Here's how the part is built. I have some questions about the finished solid (model axes, mm). Coordinates: 2 decimals unless noted, no trailing zeros. Write each loop counter-clockwise with the first axis right and the second up, starting at its lowest first coordinate (ties: lowest second). Pieces come first, ordered by that corner, then holes.
Item 1: If I drill on line 1 (Y direction, x = 2.5, z = 1.85); line 2 (Y direction, x = 13.5, z = 1.6); line 3 (X direction, y = 2.5, z = 1.85), over which ranges is the centre line in solid material (lowest first)?
Item 2: If we section it at A-A (y = 75.5): Please give me the cut outline in (x, z).
Item 3: I'm going to push flat-ended pins straight in: pin 1 Ø1.5 at (x, z) = (9, 3) entering from +Y; pin 2 Ø3 at (x, y) = (2.5, 2.5) entering from +Z. Where does each tip first touch, or does it pass through?
Item 4: If we section it at C-C (y = 54): Please give me the cut outline in (x, z).
Item 5: If we section it at B-B (x = 13.5): Please give me the cut outline in (y, z).
Item 6: If we section it at D-D (z = 2.8): Please give me the cut outline in (x, y).
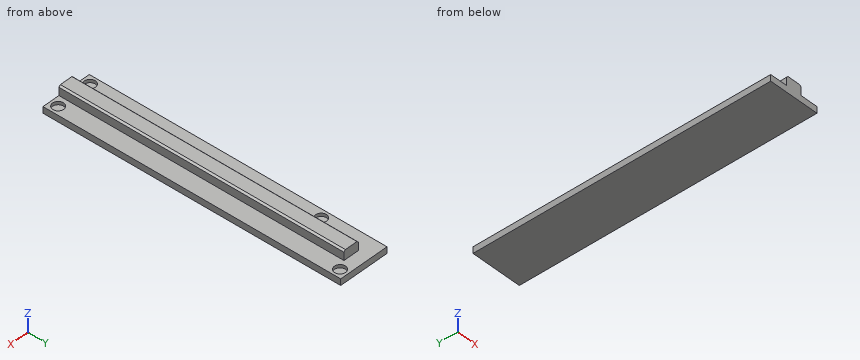
Autodesk Fusion 360 part; units mm, degrees
sketch "3D-printed conduit top outline" plane through (0, 0, 0) normal (0, 1, 0) x (1, 0, 0)
  line L0 (0, 0) -> (16, 0)
  line L1 (16, 0) -> (16, -2)
  line L2 (16, -2) -> (0, -2)
  line L3 (0, -2) -> (0, 0)
  dimension "d7" = 16
  dimension "d8" = 2
extrude "Extrude1" add sketch "3D-printed conduit top outline" along normal blind 94
sketch "Magnet holes" plane through (0, 0, 2) normal (0, 0, 1) x (-1, 0, 0)
  line L0 (0, 0) -> (-16, 0)
  line L1 (-16, 0) -> (-16, -94)
  line L2 (-16, -94) -> (0, -94)
  line L3 (0, -94) -> (0, 0)
  circle A0 centre (-2.5, -2.5) radius 2.5
  circle A1 centre (-13.5, -2.5) radius 2.5
  circle A2 centre (-2.5, -2.5) radius 1.75
  circle A3 centre (-13.5, -2.5) radius 1.75
  circle A4 centre (-2.5, -75.5) radius 1.75
  circle A5 centre (-2.5, -75.5) radius 2.5
  circle A6 centre (-13.5, -91.5) radius 2.5
  circle A7 centre (-13.5, -91.5) radius 1.75
  dimension "d11" = 5
  dimension "d12" = 5
  dimension "d13" = 3.5
  dimension "d14" = 3.5
  dimension "d17" = 0
  dimension "d18" = -73
  dimension "d32" = 0
  dimension "d33" = -89
extrude "Extrude4" cut sketch "Magnet holes" against normal blind 1 contours A2 | A3 | A4 | A7
sketch "Support rib" plane through (0, 0, 2) normal (0, 0, 1) x (-1, 0, 0)
  circle A0 centre (-13.5, -2.5) radius 1.75
  circle A1 centre (-2.5, -75.5) radius 1.75
  circle A2 centre (-2.5, -2.5) radius 1.75
  circle A3 centre (-13.5, -91.5) radius 1.75
  line L0 (0, 0) -> (-16, 0)
  line L1 (-16, 0) -> (-16, -94)
  line L2 (-16, -94) -> (0, -94)
  line L3 (0, -94) -> (0, 0)
  line L4 (-5.5, 0) -> (-10.5, 0)
  line L5 (-10.5, 0) -> (-10.5, -90)
  line L6 (-10.5, -90) -> (-5.5, -90)
  line L7 (-5.5, -90) -> (-5.5, 0)
  dimension "d36" = 5
  dimension "d37" = 5.5
  dimension "d38" = 5.5
  dimension "d39" = 4
extrude "Extrude3" add sketch "Support rib" along normal blind 3 contours L0 L4 L5 L6 L7
chamfer "Chamfer2" distance 0.5 angle 45 2 edges at (10.5, 45, 5) (5.5, 45, 5)
equation "conduit_length = 94 mm"
equation "conduit_width = 16 mm"
equation "conduit_wall_thickness = 2 mm"
equation "magnet_diameter = 3 mm"
equation "magnet_height = 1 mm"
equation "d7 = conduit_width"
equation "d8 = conduit_wall_thickness"
equation "d9 = conduit_length"
equation "d11 = magnet_diameter + 2 mm"
equation "d12 = magnet_diameter + 2 mm"
equation "d13 = magnet_diameter + 0.5 mm"
equation "d14 = magnet_diameter + 0.5 mm"
equation "d18 = -conduit_length + ( magnet_diameter + 2 mm ) + ( conduit_width )"
equation "rib_width = 5 mm"
equation "rib_height = 3 mm"
equation "d26 = rib_height"
equation "rib_chamfer = 0.5 mm"
equation "d33 = -conduit_length + ( magnet_diameter + 2 mm )"
equation "d36 = rib_width"
equation "d37 = ( conduit_width - rib_width ) / 2"
equation "d39 = 2 * conduit_wall_thickness"
equation "d40 = rib_chamfer"
Answer list:
1. line 1: y = 0 to 0.75, 4.25 to 73.75, 77.25 to 94
1. line 2: y = 0 to 0.75, 4.25 to 89.75, 93.25 to 94
1. line 3: x = 0 to 0.75, 4.25 to 11.75, 15.25 to 16
2. outline: (0, 0) - (16, 0) - (16, 2) - (10.5, 2) - (10.5, 4.5) - (10, 5) - (6, 5) - (5.5, 4.5) - (5.5, 2) - (4.25, 2) - (4.25, 1) - (0.75, 1) - (0.75, 2) - (0, 2) - close
3. pin 1: stops at y = 90
3. pin 2: stops at z = 1
4. outline: (0, 0) - (16, 0) - (16, 2) - (10.5, 2) - (10.5, 4.5) - (10, 5) - (6, 5) - (5.5, 4.5) - (5.5, 2) - (0, 2) - close
5. outline: (0, 0) - (94, 0) - (94, 2) - (93.25, 2) - (93.25, 1) - (89.75, 1) - (89.75, 2) - (4.25, 2) - (4.25, 1) - (0.75, 1) - (0.75, 2) - (0, 2) - close
6. outline: (5.5, 0) - (10.5, 0) - (10.5, 90) - (5.5, 90) - close
